Geometry check sheet. Reference: the model listing, model coordinates, mm. Face numbers are marked on the shaded views. A direction names the side the tool comes from. Give positions to 0.01 mm unless a question says otherwise; leave off trailing zeros. Write each loop counter-clockwise with the first axis right and the second up, starting at its lowest first coordinate (ties: lowest second). Pieces come first, ordered by that corner, then holes. Notation, with made-up numbers: M 19.5,31 L 37.5,31 A17 ccw 37.5,53 Z; hole C 18.25,-6 d3. An arc over 180 degrees is marked long. Use one line per item in the form item = value. Start each with the question number.
```python
from build123d import *

# Parameters (mm, degrees)
F1_DEPTH = 60


with BuildPart() as f1:
    # F0 (on Front) → F1 (new body)
    with BuildSketch(Plane.XZ):
        with BuildLine():
            Line((19, 1.732051), (1.18418, 32.589956))
            ThreePointArc((1.18418, 32.589956), (0.194399, 33.082269), (-0.644148, 32.361937))
            Line((-0.644148, 32.361937), (-9.790771, 0))
            Line((-9.790771, 0), (-7.40067, 0))
            Line((-7.40067, 0), (0.011709, 26.225959))
            ThreePointArc((0.011709, 26.225959), (0.850256, 26.946291), (1.840037, 26.453979))
            Line((1.840037, 26.453979), (17.113249, 0))
            Line((17.113249, 0), (20, 0))
            Line((20, 0), (19, 1.732051))
        make_face()
        with BuildLine():
            Line((27.660254, 6.732051), (19, 1.732051))
            Line((19, 1.732051), (20, 0))
            Line((20, 0), (28.660254, 5))
            ThreePointArc((28.660254, 5), (29.12618, 5.607206), (29.026279, 6.366025))
            Line((29.026279, 6.366025), (27.454006, 9.089284))
            Line((27.454006, 9.089284), (25.160254, 11.062178))
            Line((25.160254, 11.062178), (27.660254, 6.732051))
        make_face()
    extrude(amount=F1_DEPTH)


solid = f1.part
```
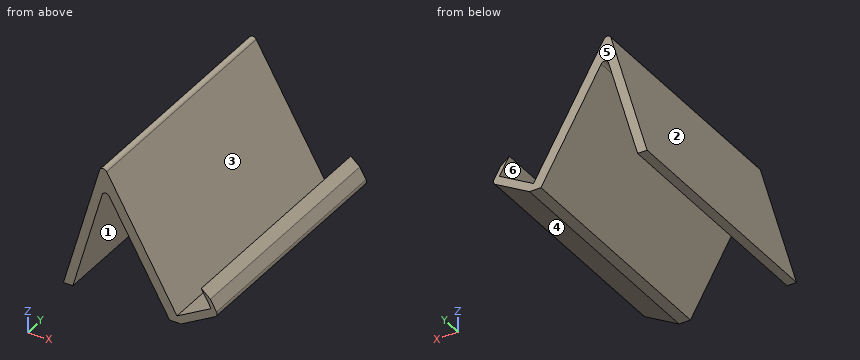
(1) Thickness scan on probe 1 along X at (y, z) = (-53, 10.5); probe 2 along X at (y, z) = (-22, 12.5); probe 3 along X at (y, z) = (-51.5, 24.5). Record the ranges inside material, lowest first. Write a range as [from, to].
(2) Sectioned sample at B-B, the plane z = 12.5. Record the boundary of the cut face in (x, y), plus the area to 3 significant figures.
(3) Depth check by flat-ended pin: pin 1 (6 mm diameter, centred on y = -53.5, z = 15.5, fed in from +X); pin 2 (6 mm diameter, centred on x = 3, y = -17, fed in from +Z); pin 3 (8 mm diameter, centred on x = 4, z = 9.5, fed in from +Y); pin 4 (1 mm diameter, centred on x = -0.5, y = -44.5, fed in from +Z). Enter the tip coordinate at first touch or a pass-through.
(4) Sectioned sample at C-C, the plane z = 30. Record the boundary of the cut face in (x, y).
(5) Draft check along X on the marked faces 4, 5 and 6. Enter one of: released by +X, released by -X, zero draft, split by the parting line, or undercut.
(6) Sectioned sample at A-A, the plane y = -54.5. Record the boundary of the cut face in (x, z).
(7) Tool access check on the marked faces 1, 2 and 3. Record the directions out of +Z, -Z, +X, -X, +Y, -Y that give a thin tool (end or side, any length) a straight path to the whole face; none if there is none.
(8) Sectioned sample at D-D, the plane x = 14. Record the boundary of the cut face in (y, z).
Numbers:
q1.probe_1 = [-6.82, -4.43], [11.05, 13.94], [25.48, 25.81]
q1.probe_2 = [-6.26, -3.87], [9.9, 12.78]
q1.probe_3 = [-2.87, -0.48], [2.97, 5.85]
q2.outline = M -6.26,-60 L -3.87,-60 L -3.87,0 L -6.26,0 Z; M 9.9,-60 L 12.78,-60 L 12.78,0 L 9.9,0 Z
q2.area = 317 mm2
q3.pin_1 = 12.78
q3.pin_2 = 33.09
q3.pin_3 = through
q3.pin_4 = 33.04
q4.outline = M -1.31,-60 L 2.68,-60 L 2.68,0 L -1.31,0 Z
q5.face_4 = released by +X
q5.face_5 = zero draft
q5.face_6 = undercut
q6.outline = M -9.79,0 L -7.4,0 L 0.01,26.23 A1 cw 1.84,26.45 L 17.11,0 L 20,0 L 28.66,5 A1 ccw 29.03,6.37 L 27.45,9.09 L 25.16,11.06 L 27.66,6.73 L 19,1.73 L 1.18,32.59 A1 ccw -0.64,32.36 Z
q7.face_1 = -Z, +Y, -Y
q7.face_2 = +Z, -X, +Y, -Y
q7.face_3 = +Z, +Y, -Y
q8.outline = M -60,5.39 L 0,5.39 L 0,10.39 L -60,10.39 Z
